For this review, take the finished solid that the model builds, in its own axes (mm). A direction names the side the tool comes from. Give positions to 0.01 mm unless a question says otherwise; leave off trailing zeros. Loops run counter-clockwise (first coordinate to the right, second up) from the corner with the lowest first, then second, coordinate; pieces in that order, holes last. Notation, with made-up numbers: (28, -22.5) -> (70, -22.5) arc R19 cw to (70, -9.5) -> close; hole circle Ø11 at (30.25, -24). An arc over 180 degrees is marked (long way). Answer as CSV lines item,"result". Start each with the question number.
Item 1: Add section A-A on y = -15. State the section outline as (x, z) points.
Item 2: Clearance check with flat-ended pins moving along their axes: P1, Ø3.5, axis at y = 7.5, z = 13.5, coming from the -X side; P2, Ø4, axis at y = 26.3, z = -4, coming from the +X side; P3, Ø2.5, axis at x = 8, y = -5, coming from the +Z side. State where each tip first meets the part, or that it passes through.
Item 3: For L1, parallel to Y at x = -6.15, z = 13; L2, parallel to X at y = -6, z = 12; L3, parallel to X at y = 6.5, z = 16, list the stretches that pass through material, from the lowest coordinate up. Write a range as from..to.
Item 4: Machinability: for faces 1 (the face through (-3, 8, 13)), 2 (the face through (-7, 8, 16)), 3 (the face through (4.5, 4, 18)), 4 (the face through (-10, 2, -6)), which of the approach directions +Z, -Z, +X, -X, +Y, -Y give a long, thin tool a straight path to every point of the face, cutting with its end or side? Answer none if there is none.
Item 5: The part is to be moulded in two halves that separate along Y. For faces 5 (the face through (-8.622, -8.92, 10.586)), 6 (the face through (-12, 28.8, -9)), 7 (the face through (9, -20, 8)), say which applies: +Y half, -Y half, draft (parallel to the pull), parting line (faces both ways), or undercut.
```python
from build123d import *

# Parameters (mm, degrees)
BOSS_EXTRUDE1_DEPTH      = 37
BOSS_EXTRUDE1_DEPTH_BACK = 20
CUT_EXTRUDE5_DEPTH       = 7
CHAMFER2_SIZE            = 3.5
CHAMFER3_SIZE            = 0.5
SKETCH6_R                = 1.55
CUT_EXTRUDE6_DEPTH       = 10
CUT_EXTRUDE7_START       = -2.8
CUT_EXTRUDE7_DEPTH       = 3.2
CUT_EXTRUDE9_DEPTH       = 10
BOSS_EXTRUDE2_DEPTH      = 3
SKETCH10_W               = 7
SKETCH10_H               = 8.2
CUT_EXTRUDE10_DEPTH      = 4
SKETCH11_R               = 1.25
CUT_EXTRUDE11_DEPTH      = 4
CHAMFER4_SIZE            = 3
CUT_EXTRUDE12_DEPTH      = 9
CHAMFER5_SIZE            = 1
SKETCH14_W               = 3.4
SKETCH14_H               = 10.5
CUT_EXTRUDE13_DEPTH      = 3
CHAMFER6_SIZE            = 1
CHAMFER7_SIZE            = 0.4
CHAMFER7_SIZE2           = 1


# Some blends are built 0.0001 mm under size
with BuildPart() as part:
    # Sketch2 → Boss-Extrude1 (new, two sides: drawn at the far end of the back side and taken through both)
    with BuildSketch(Plane(origin=(0, 0, 0), x_dir=(1, 0, 0), z_dir=(0, 1, 0)).offset(-BOSS_EXTRUDE1_DEPTH_BACK)):
        with BuildLine():
            Line((10.05, -12.9), (4.5, -12.9))
            Line((4.5, -12.9), (4.5, -20))
            Line((4.5, -20), (-13, -20))
            Line((-13, -20), (-13, 11))
            Line((-13, 11), (-4, 11))
            Line((-4, 11), (-4, 9.816312953))
            ThreePointArc((-4, 9.816312953), (-7.25402814, -7.729105754), (10.05, -3.37008902))
            Line((10.05, -3.37008902), (10.05, -12.9))
        make_face()
    extrude(amount=BOSS_EXTRUDE1_DEPTH + BOSS_EXTRUDE1_DEPTH_BACK)

    # Sketch5 → Cut-Extrude5 (cut)
    with BuildSketch(Plane(origin=(4.5, 0, 0), x_dir=(0, 0, -1), z_dir=(1, 0, 0))):
        Polygon((-15.8, 5.718), (-15.3, 6.218), (-15.3, 6.718), (-15.8, 7.218), (-15.8, 7.75), (-15.3, 8.25), (-15.3, 8.75), (-15.8, 9.25), (-15.8, 9.782), (-15.3, 10.282), (-15.3, 10.782), (-15.8, 11.282), (-15.8, 14.5), (-16.3, 15.366025404), (-16.3, 37), (-14.3, 37), (-14.3, -20), (-16.3, -20), (-16.3, 1.633974596), (-15.8, 2.5), align=None)
    extrude(amount=-CUT_EXTRUDE5_DEPTH, mode=Mode.SUBTRACT)

    # Chamfer2
    # the kernel refuses this chamfer: 3.5 mm, written as the material it takes off along each edge
    with BuildSketch(Plane(origin=(19.050890458, -20, 12.9), x_dir=(0, 0.9996219169112968, 0.02749587661058662), z_dir=(-1, 0, 0))) as chamfer2_piece_1:
        Polygon((CHAMFER2_SIZE * 0.999621916911, CHAMFER2_SIZE * 0.0274958766106), (-CHAMFER2_SIZE * 0.0274958766106, CHAMFER2_SIZE * 0.999621916911), (0, 0), align=None)
    extrude(amount=14.550890458, mode=Mode.SUBTRACT)

    # Chamfer3
    # the kernel refuses this chamfer: 0.5 mm, written as the material it takes off along each edge
    with BuildSketch(Plane(origin=(-4, -20, -12.285841494), x_dir=(-0.9996219169112968, -0.0274958766105891, 0), z_dir=(0, 0, 1))) as chamfer3_piece_1:
        Polygon((CHAMFER3_SIZE * 0.999621916911, -CHAMFER3_SIZE * 0.0274958766106), (-CHAMFER3_SIZE * 0.0274958766106, -CHAMFER3_SIZE * 0.999621916911), (0, 0), align=None)
    extrude(amount=3.755370035, mode=Mode.SUBTRACT)
    with BuildSketch(Plane(origin=(0, -20, 0), x_dir=(-0.26232896064226713, 0, -0.9649785056716795), z_dir=(0.9649785056716795, 0, -0.26232896064226713))) as chamfer3_piece_2:
        Polygon((10.6 + CHAMFER3_SIZE, 0), (10.6, CHAMFER3_SIZE), (10.6, 0), align=None)
    revolve(axis=Axis((0, -20, 0), (0, 1, 0)), revolution_arc=196.87436844, mode=Mode.SUBTRACT)
    with BuildSketch(Plane(origin=(5.785841494, -20, 14.3), x_dir=(0, -0.0274958766105891, -0.9996219169112968), z_dir=(-1, 0, 0))) as chamfer3_piece_3:
        Polygon((CHAMFER3_SIZE * 0.999621916911, -CHAMFER3_SIZE * 0.0274958766106), (-CHAMFER3_SIZE * 0.0274958766106, -CHAMFER3_SIZE * 0.999621916911), (0, 0), align=None)
    extrude(amount=8.285841494, mode=Mode.SUBTRACT)
    with BuildSketch(Plane(origin=(-2.5, -20, 14.3), x_dir=(-0.9996219169112968, -0.027495876610589075, 0), z_dir=(0, 0, 1))) as chamfer3_piece_4:
        Polygon((CHAMFER3_SIZE * 0.999621916911, -CHAMFER3_SIZE * 0.0274958766106), (-CHAMFER3_SIZE * 0.0274958766106, -CHAMFER3_SIZE * 0.999621916911), (0, 0), align=None)
    extrude(amount=2, mode=Mode.SUBTRACT)
    with BuildSketch(Plane(origin=(5.785841494, -20, 16.3), x_dir=(0, -0.027495876610589005, 0.9996219169112968), z_dir=(-1, 0, 0))) as chamfer3_piece_5:
        Polygon((CHAMFER3_SIZE * 0.999621916911, CHAMFER3_SIZE * 0.0274958766106), (-CHAMFER3_SIZE * 0.0274958766106, CHAMFER3_SIZE * 0.999621916911), (0, 0), align=None)
    extrude(amount=8.285841494, mode=Mode.SUBTRACT)
    with BuildSketch(Plane(origin=(4.5, -20, 15.014158506), x_dir=(-0.9996219169112968, -0.027495876610589075, 0), z_dir=(0, 0, 1))) as chamfer3_piece_6:
        Polygon((CHAMFER3_SIZE * 0.999621916911, -CHAMFER3_SIZE * 0.0274958766106), (-CHAMFER3_SIZE * 0.0274958766106, -CHAMFER3_SIZE * 0.999621916911), (0, 0), align=None)
    extrude(amount=6.271682988, mode=Mode.SUBTRACT)
    with BuildSketch(Plane(origin=(5.785841494, -20, 20), x_dir=(0, -0.027495876610589005, -0.9996219169112968), z_dir=(-1, 0, 0))) as chamfer3_piece_7:
        Polygon((CHAMFER3_SIZE * 0.999621916911, -CHAMFER3_SIZE * 0.0274958766106), (-CHAMFER3_SIZE * 0.0274958766106, -CHAMFER3_SIZE * 0.999621916911), (0, 0), align=None)
    extrude(amount=20.071682988, mode=Mode.SUBTRACT)
    with BuildSketch(Plane(origin=(-13, -20, 21.285841494), x_dir=(0.9996219169112968, -0.0274958766105891, 0), z_dir=(0, 0, -1))) as chamfer3_piece_8:
        Polygon((CHAMFER3_SIZE * 0.999621916911, -CHAMFER3_SIZE * 0.0274958766106), (-CHAMFER3_SIZE * 0.0274958766106, -CHAMFER3_SIZE * 0.999621916911), (0, 0), align=None)
    extrude(amount=33.571682988, mode=Mode.SUBTRACT)
    with BuildSketch(Plane(origin=(-14.285841494, -20, -11), x_dir=(0, -0.0274958766105891, 0.9996219169112968), z_dir=(1, 0, 0))) as chamfer3_piece_9:
        Polygon((CHAMFER3_SIZE * 0.999621916911, -CHAMFER3_SIZE * 0.0274958766106), (-CHAMFER3_SIZE * 0.0274958766106, -CHAMFER3_SIZE * 0.999621916911), (0, 0), align=None)
    extrude(amount=11.571682988, mode=Mode.SUBTRACT)
    with BuildSketch(Plane(origin=(0, -20, 0), x_dir=(0.3514513132600512, 0, 0.9362061602060656), z_dir=(-0.9362061602060656, 0, 0.3514513132600512))) as chamfer3_piece_10:
        Polygon((10.6 + CHAMFER3_SIZE, 0), (10.6, CHAMFER3_SIZE), (10.6, 0), align=None)
    revolve(axis=Axis((0, -20, 0), (0, 1, 0)), revolution_arc=57.836903019, mode=Mode.SUBTRACT)
    with BuildSketch(Plane(origin=(5.785841494, -20, 14.3), x_dir=(0, -0.0274958766105891, -0.9996219169112968), z_dir=(-1, 0, 0))) as chamfer3_piece_11a_section:
        Polygon((CHAMFER3_SIZE * 0.999621916911, -CHAMFER3_SIZE * 0.0274958766106), (-CHAMFER3_SIZE * 0.0274958766106, -CHAMFER3_SIZE * 0.999621916911), (0, 0), align=None)
    chamfer3_piece_11a = extrude(amount=9.571682988, mode=Mode.PRIVATE)
    chamfer3_piece_11a = split(chamfer3_piece_11a, bisect_by=Plane(origin=(-2.5, -19.835103187, 14.135103187), z_dir=(-1, 0, 0)), keep=Keep.TOP, mode=Mode.PRIVATE)
    with BuildSketch(Plane(origin=(-2.5, -20, 13.014158506), x_dir=(-0.9996219169112968, -0.027495876610589075, 0), z_dir=(0, 0, 1))) as chamfer3_piece_11b_section:
        Polygon((CHAMFER3_SIZE * 0.999621916911, -CHAMFER3_SIZE * 0.0274958766106), (-CHAMFER3_SIZE * 0.0274958766106, -CHAMFER3_SIZE * 0.999621916911), (0, 0), align=None)
    chamfer3_piece_11b = extrude(amount=3.285841494, mode=Mode.PRIVATE)
    chamfer3_piece_11b = split(chamfer3_piece_11b, bisect_by=Plane(origin=(-2.664896813, -19.835103187, 14.3), z_dir=(0, 0, -1)), keep=Keep.TOP, mode=Mode.PRIVATE)
    chamfer3_piece_11 = chamfer3_piece_11a & chamfer3_piece_11b
    add(chamfer3_piece_11, mode=Mode.SUBTRACT)
    with BuildSketch(Plane(origin=(-2.5, -20, 14.3), x_dir=(-0.9996219169112968, -0.027495876610589075, 0), z_dir=(0, 0, 1))) as chamfer3_piece_12a_section:
        Polygon((CHAMFER3_SIZE * 0.999621916911, -CHAMFER3_SIZE * 0.0274958766106), (-CHAMFER3_SIZE * 0.0274958766106, -CHAMFER3_SIZE * 0.999621916911), (0, 0), align=None)
    chamfer3_piece_12a = extrude(amount=3.285841494, mode=Mode.PRIVATE)
    chamfer3_piece_12a = split(chamfer3_piece_12a, bisect_by=Plane(origin=(-2.664896813, -19.835103187, 16.3), z_dir=(0, 0, 1)), keep=Keep.TOP, mode=Mode.PRIVATE)
    with BuildSketch(Plane(origin=(5.785841494, -20, 16.3), x_dir=(0, -0.027495876610589005, 0.9996219169112968), z_dir=(-1, 0, 0))) as chamfer3_piece_12b_section:
        Polygon((CHAMFER3_SIZE * 0.999621916911, CHAMFER3_SIZE * 0.0274958766106), (-CHAMFER3_SIZE * 0.0274958766106, CHAMFER3_SIZE * 0.999621916911), (0, 0), align=None)
    chamfer3_piece_12b = extrude(amount=9.571682988, mode=Mode.PRIVATE)
    chamfer3_piece_12b = split(chamfer3_piece_12b, bisect_by=Plane(origin=(-2.5, -19.835103187, 16.464896813), z_dir=(-1, 0, 0)), keep=Keep.TOP, mode=Mode.PRIVATE)
    chamfer3_piece_12 = chamfer3_piece_12a & chamfer3_piece_12b
    add(chamfer3_piece_12, mode=Mode.SUBTRACT)

    # Sketch6 → Cut-Extrude6 (cut)
    with BuildSketch(Plane.ZY.offset(13)):
        with Locations((13, 7.5)):
            Circle(SKETCH6_R)
        with Locations((13, -7.5)):
            Circle(SKETCH6_R)
    extrude(amount=-CUT_EXTRUDE6_DEPTH, mode=Mode.SUBTRACT)

    # Sketch7 → Cut-Extrude7 (cut)
    with BuildSketch(Plane.ZY.offset(13).offset(CUT_EXTRUDE7_START)):
        Polygon((21.967267325, -4.7), (21.967267325, -10.3), (11.383419246, -10.3), (9.766838493, -7.5), (11.383419246, -4.7), align=None)
        Polygon((11.383419246, 4.7), (9.559772236, 7.5), (11.383419246, 10.3), (21.967267325, 10.3), (21.967267325, 4.7), align=None)
    extrude(amount=-CUT_EXTRUDE7_DEPTH, mode=Mode.SUBTRACT)

    # Sketch9 → Cut-Extrude9 (cut)
    with BuildSketch(Plane.ZY.offset(13)):
        Polygon((-11, 28), (-6, 23), (-6, -20), (-11, -20), align=None)
    extrude(amount=-CUT_EXTRUDE9_DEPTH, mode=Mode.SUBTRACT)

    # Sketch12 → Boss-Extrude2 (add)
    with BuildSketch(Plane.ZY.offset(13)):
        Polygon((9, 37), (9, 22.951792944), (-5.951792944, 22.951792944), (-11, 28), (-11, 37), align=None)
    extrude(amount=BOSS_EXTRUDE2_DEPTH)

    # Sketch10 → Cut-Extrude10 (cut)
    with BuildSketch(Plane(origin=(0, 0, -11), x_dir=(-1, 0, 0), z_dir=(0, 0, -1))):
        with Locations((12.5, 32.9)):
            Rectangle(SKETCH10_W, SKETCH10_H)
    extrude(amount=-CUT_EXTRUDE10_DEPTH, mode=Mode.SUBTRACT)

    # Sketch11 → Cut-Extrude11 (cut)
    with BuildSketch(Plane.ZY.offset(16)):
        with Locations((-4, 26.3)):
            Circle(SKETCH11_R)
        with Locations((6, 26.3)):
            Circle(SKETCH11_R)
    extrude(amount=-CUT_EXTRUDE11_DEPTH, mode=Mode.SUBTRACT)

    # Chamfer4
    chamfer4_edges = [part.edges().sort_by_distance(p)[0] for p in [
        (-13, 29.975896472, 9),
        (-13, 22.951792944, 1.524103528),
    ]]
    chamfer(chamfer4_edges, length=CHAMFER4_SIZE - 0.0001)  # a hair under: the kernel refuses the full size

    # Sketch13 → Cut-Extrude12 (cut)
    with BuildSketch(Plane(origin=(0, 37, 0), x_dir=(1, 0, 0), z_dir=(0, 1, 0))):
        Polygon((-16, -9), (0, -9), (0, 6.411173943), (12, 6.411173943), (12, -20), (-16, -20), align=None)
    extrude(amount=-CUT_EXTRUDE12_DEPTH, mode=Mode.SUBTRACT)

    # Chamfer5
    chamfer5_edges = [part.edges().sort_by_distance(p)[0] for p in [
        (-10.8, 37, 9),
    ]]
    chamfer(chamfer5_edges, length=CHAMFER5_SIZE)

    # Sketch14 → Cut-Extrude13 (cut)
    with BuildSketch(Plane.XY.offset(12.9)):
        with Locations((7.25, -5.25)):
            Rectangle(SKETCH14_W, SKETCH14_H)
    extrude(amount=-CUT_EXTRUDE13_DEPTH, mode=Mode.SUBTRACT)

    # Chamfer6
    chamfer6_edges = [part.edges().sort_by_distance(p)[0] for p in [
        (-13, 1.75, -6),
    ]]
    chamfer(chamfer6_edges, length=CHAMFER6_SIZE)

    # Chamfer7
    chamfer7_edges = [part.edges().sort_by_distance(p)[0] for p in [
        (4.5, 4.25, 14.3),
    ]]
    chamfer7_side = [part.faces().sort_by_distance(p)[0] for p in [
        (4.5, 2.170208938, 13.449589105),
    ]]
    chamfer(chamfer7_edges, length=CHAMFER7_SIZE, length2=CHAMFER7_SIZE2, reference=chamfer7_side[0])


solid = part.part
```
Computed values:
1,outline,"(-13, -5) -> (-12, -6) -> (-8.74, -6) arc R10.6 cw (long way) to (10.05, 3.37) -> (10.05, 12.9) -> (4.5, 12.9) -> (4.5, 13.9) -> (3.5, 14.3) -> (-2.5, 14.3) -> (-2.5, 16.3) -> (4.5, 16.3) -> (4.5, 20) -> (-13, 20) -> close"
2,P1,"x = -13"
2,P2,"x = -8.74"
2,P3,"z = 12.9"
3,L1,"-20..-9.05, -5.95..5.95, 9.05..28"
3,L2,"-13..-10.2, -7..5.55, 8.95..10.05"
3,L3,"-13..-10.2, -7..4.5"
4,face 1,"-X"
4,face 2,"+Z"
4,face 3,"+Z, +X, +Y, -Y"
4,face 4,"-Z, +X, -X, -Y"
5,face 5,"undercut"
5,face 6,"+Y half"
5,face 7,"-Y half"
